Work out the finished part from the listing and answer in its coordinate system (mm). A direction names the side the tool comes from. Coordinates: 2 decimals unless noted, no trailing zeros. Loops run counter-clockwise (first coordinate to the right, second up) from the corner with the lowest first, then second, coordinate; pieces in that order, holes last. Notation, with made-up numbers: (64.25, 48.5) -> (84.25, 48.5) arc R15 ccw to (84.25, 73.5) -> close; hole circle Ø1 at (83.5, -14.5). An arc over 180 degrees is marked (long way). Use a Markdown table: item, result.
from build123d import *

# Parameters (mm, degrees)
SKETCH_2_W          = 132
SKETCH_2_H          = 200
EXTRUDE_1_DEPTH     = 6
SKETCH_3_R          = 57.15
CUT_EXTRUDE_1_DEPTH = 6
EXTRUDE_START       = 3
SKETCH_6_R          = 57.15
SKETCH_6_R_2        = 55.15
EXTRUDE_2_DEPTH     = 3
SKETCH_10_R         = 1.6
CUT_EXTRUDE_2_DEPTH = 6
SKETCH_11_R         = 13
CUT_EXTRUDE_3_DEPTH = 6
SKETCH_12_R         = 16
CUT_EXTRUDE_4_DEPTH = 2.6
SKETCH_13_R         = 4.2
CUT_EXTRUDE_5_DEPTH = 2.6
FILLET_1_R          = 2
SKETCH_14_R         = 2.25
CUT_EXTRUDE_6_DEPTH = 6
FILLET_2_R          = 6
SKETCH_15_R         = 1.6
CUT_EXTRUDE_7_DEPTH = 6
SKETCH_17_R         = 15
CUT_EXTRUDE_9_DEPTH = 6


with BuildPart() as part:
    # 草图2 → 凸台-拉伸1 (new body)
    with BuildSketch(Plane(origin=(0, 0, 0), x_dir=(1, 0, 0), z_dir=(0, 1, 0))):
        Rectangle(SKETCH_2_W, SKETCH_2_H)
    extrude(amount=EXTRUDE_1_DEPTH)

    # 草图3 → 切除-拉伸1 (cut)
    with BuildSketch(Plane(origin=(0, 6, 0), x_dir=(1, 0, 0), z_dir=(0, 1, 0))):
        with Locations(Location((0, 34, 0), (0, 0, 270))):
            Circle(SKETCH_3_R)
    extrude(amount=-CUT_EXTRUDE_1_DEPTH, mode=Mode.SUBTRACT)

    # 草图6 → 凸台-拉伸2 (add)
    with BuildSketch(Plane(origin=(0, 0, 0), x_dir=(1, 0, 0), z_dir=(0, 1, 0)).offset(EXTRUDE_START)):
        with Locations(Location((0, 34, 0), (0, 0, 270))):
            Circle(SKETCH_6_R)
        with Locations(Location((0, 34, 0), (0, 0, 270))):
            Circle(SKETCH_6_R_2, mode=Mode.SUBTRACT)
    extrude(amount=-EXTRUDE_2_DEPTH)

    # 草图10 → 切除-拉伸2 (cut)
    with BuildSketch(Plane(origin=(0, 6, 0), x_dir=(1, 0, 0), z_dir=(0, 1, 0))):
        with Locations(Location((43.133513652, -9.133513652, 0), (0, 0, 270))):
            Circle(SKETCH_10_R)
        with Locations(Location((-43.133513652, -9.133513652, 0), (0, 0, 270))):
            Circle(SKETCH_10_R)
        with Locations(Location((-43.133513652, 77.133513652, 0), (0, 0, 270))):
            Circle(SKETCH_10_R)
        with Locations(Location((43.133513652, 77.133513652, 0), (0, 0, 270))):
            Circle(SKETCH_10_R)
    extrude(amount=-CUT_EXTRUDE_2_DEPTH, mode=Mode.SUBTRACT)

    # 草图11 → 切除-拉伸3 (cut)
    with BuildSketch(Plane(origin=(0, 6, 0), x_dir=(1, 0, 0), z_dir=(0, 1, 0))):
        with Locations(Location((0, -64, 0), (0, 0, 270))):
            Circle(SKETCH_11_R)
    extrude(amount=-CUT_EXTRUDE_3_DEPTH, mode=Mode.SUBTRACT)

    # 草图12 → 切除-拉伸4 (cut)
    with BuildSketch(Plane(origin=(0, 6, 0), x_dir=(1, 0, 0), z_dir=(0, 1, 0))):
        with Locations(Location((0, -64, 0), (0, 0, 270))):
            Circle(SKETCH_12_R)
    extrude(amount=-CUT_EXTRUDE_4_DEPTH, mode=Mode.SUBTRACT)

    # 草图13 → 切除-拉伸5 (cut)
    with BuildSketch(Plane(origin=(0, 6, 0), x_dir=(1, 0, 0), z_dir=(0, 1, 0))):
        with Locations((0, -44.75)):
            Circle(SKETCH_13_R)
    extrude(amount=-CUT_EXTRUDE_5_DEPTH, mode=Mode.SUBTRACT)

    # 圆角1
    fillet_1_edges = [part.edges().sort_by_distance(p)[0] for p in [
        (2.418429967, 4.7, 48.183831169),
        (-2.418429967, 4.7, 48.183831169),
    ]]
    fillet(fillet_1_edges, radius=FILLET_1_R)

    # 草图14 → 切除-拉伸6 (cut)
    with BuildSketch(Plane(origin=(0, 6, 0), x_dir=(1, 0, 0), z_dir=(0, 1, 0))):
        with Locations(Location((0, -35, 0), (0, 0, 270))):
            Circle(SKETCH_14_R)
        with Locations(Location((25.11473671, -78.5, 0), (0, 0, 270))):
            Circle(SKETCH_14_R)
        with Locations(Location((-25.11473671, -78.5, 0), (0, 0, 270))):
            Circle(SKETCH_14_R)
    extrude(amount=-CUT_EXTRUDE_6_DEPTH, mode=Mode.SUBTRACT)

    # 圆角2
    fillet_2_edges = [part.edges().sort_by_distance(p)[0] for p in [
        (66, 3, 100),
        (-66, 3, 100),
        (-66, 3, -100),
        (66, 3, -100),
    ]]
    fillet(fillet_2_edges, radius=FILLET_2_R)

    # 草图15 → 切除-拉伸7 (cut)
    with BuildSketch(Plane(origin=(0, 6, 0), x_dir=(1, 0, 0), z_dir=(0, 1, 0))):
        with Locations(Location((60, 94, 0), (0, 0, 270))):
            Circle(SKETCH_15_R)
        with Locations(Location((-60, 94, 0), (0, 0, 90))):
            Circle(SKETCH_15_R)
        with Locations(Location((60, -94, 0), (0, 0, 90))):
            Circle(SKETCH_15_R)
        with Locations(Location((-60, -94, 0), (0, 0, 270))):
            Circle(SKETCH_15_R)
        with Locations(Location((60, 0, 0), (0, 0, 270))):
            Circle(SKETCH_15_R)
        with Locations(Location((-60, 0, 0), (0, 0, 90))):
            Circle(SKETCH_15_R)
    extrude(amount=-CUT_EXTRUDE_7_DEPTH, mode=Mode.SUBTRACT)

    # 草图17 → 切除-拉伸9 (cut)
    with BuildSketch(Plane(origin=(0, 6, 0), x_dir=(1, 0, 0), z_dir=(0, 1, 0))):
        with Locations(Location((34.641016151, -44, 0), (0, 0, 270))):
            Circle(SKETCH_17_R)
        with Locations(Location((-34.641016151, -44, 0), (0, 0, 90))):
            Circle(SKETCH_17_R)
    extrude(amount=-CUT_EXTRUDE_9_DEPTH, mode=Mode.SUBTRACT)


solid = part.part
Q1. Consider line 1 (X direction, y = 4.5, z = -94); line 2 (Z direction, x = 26.5, y = 5); line 3 (X direction, y = 1.75, z = -34). Determine where each line is inside the solid, lowest interval first. Write a range as [from, to].
Solved:
| item | result |
|---|---|
| line 1 | [-66, -61.6], [-58.4, 58.4], [61.6, 66] |
| line 2 | [-100, -84.63], [16.63, 31.4], [56.6, 76.73], [80.27, 100] |
| line 3 | [-66, -55.15], [55.15, 66] |
Q2. For faces 4 (the flat face through (4, 3.4, 51)), 5 (the flat face through (-1, 3, 100)), determine the directions among +Z, -Z, +X, -X, +Y, -Y from which every point of the face is accessible in a straight line to the end or side of a thin tool.
Solved:
| item | result |
|---|---|
| face 4 | +Y |
| face 5 | +Z, +X, -X, +Y, -Y |
Q3. Determine the mould class of faces 1 (the cylindrical face through (-25.976, 3.042, 80.578)), 2 (the cylindrical face through (64.196, 3.042, 98.289)), 3 (the flat face through (28, 6, 21)) for opening direction Z: pulls with the +Z half, pulls with the -Z half, needs draft (parallel to the pull), parting line crosses it, or undercut.
Solved:
| item | result |
|---|---|
| face 1 | undercut |
| face 2 | pulls with the +Z half |
| face 3 | needs draft |
Q4. Section D-D on z = -23.5 is taken. Determine the outline of the cut face in (x, y), and give its area (3 significant figures).
Solved:
| item | result |
|---|---|
| outline | (-66, 0) -> (-54.14, 0) -> (-54.14, 3) -> (-56.18, 3) -> (-56.18, 6) -> (-66, 6) -> close; (54.14, 0) -> (66, 0) -> (66, 6) -> (56.18, 6) -> (56.18, 3) -> (54.14, 3) -> close |
| area | 130 mm² |
Q5. Given pin 1 Ø18 at (x, z) = (34.64, 44) entering from -Y, flat-ended and moving along its own axis, determine where the tip first touches the part or whether it passes through.
Solved:
| item | result |
|---|---|
| pin 1 | through |
Q6. Section C-C on y = 2 is taken. State how many separate pieces and enclosed holes the cut face has, and give its area (3 significant figures).
Solved:
| item | result |
|---|---|
| separate pieces | 1 |
| enclosed holes | 17 |
| area | 14,700 mm² |
Q7. Section A-A on z = 64 is taken. Determine the outline of the cut face in (x, y).
Solved:
| item | result |
|---|---|
| outline | (-66, 0) -> (-13, 0) -> (-13, 3.4) -> (-16, 3.4) -> (-16, 6) -> (-66, 6) -> close; (13, 0) -> (66, 0) -> (66, 6) -> (16, 6) -> (16, 3.4) -> (13, 3.4) -> close |
Q8. Section B-B on z = 35 is taken. Determine the outline of the cut face in (x, y), and give its area (3 significant figures).
Solved:
| item | result |
|---|---|
| outline | (-66, 0) -> (-46.64, 0) -> (-46.64, 6) -> (-66, 6) -> close; (-22.64, 0) -> (-2.25, 0) -> (-2.25, 6) -> (-22.64, 6) -> close; (2.25, 0) -> (22.64, 0) -> (22.64, 6) -> (2.25, 6) -> close; (46.64, 0) -> (66, 0) -> (66, 6) -> (46.64, 6) -> close |
| area | 477 mm² |
